Verification items for this drawing (mm, ordinates from the low corner). A direction names the side the tool comes from. Round coordinates to 2 decimals unless told otherwise and drop trailing zeros. Order: outer loops, then holes, each group sorted by start corner. A loop starts at its lowest first (then second) coordinate and runs counter-clockwise, first axis right, second up.
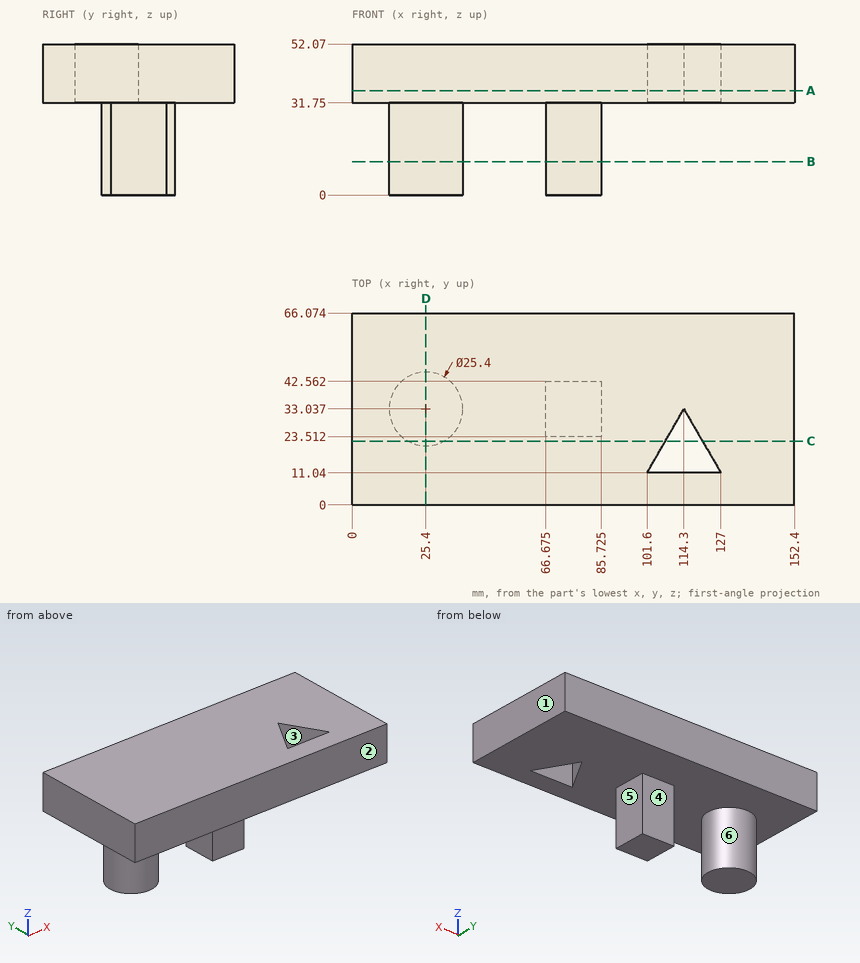
Item 1: Access from +Z, -Z, +X, -X, +Y, -Y to the whole of each face (thin tool, end or side, straight path). Record for the marked faces 4, 5 and 6.
Answer:
face 4: -Z, +X, +Y
face 5: -Z, +X, +Y, -Y
face 6: -Z
Item 2: Sectioned sample at A-A (z = 36). Record the cut outline in (x, y), and give its area (3 significant figures).
Answer:
outline: (0, 0) - (152.4, 0) - (152.4, 66.07) - (0, 66.07) - close; hole (101.6, 11.04) - (127, 11.04) - (114.3, 33.04) - close
area: 9,790 mm2
Item 3: Go/stop test with flat-tipped pins: P1, Ø9.5, axis at x = 78.5, z = 10.5, coming from the +Y side; P2, Ø10, axis at y = 47.5, z = 14.5, coming from the -X side; P3, Ø21, axis at x = 73, z = 20.5, coming from the -Y side; P4, Ø8, axis at x = 113.5, y = 23.5, coming from the +Z side. Record where each tip stops, or that it passes through.
Answer:
P1: stops at y = 42.56
P2: stops at x = 16.93
P3: stops at y = 23.51
P4: passes through
Item 4: Release check for a two-part mould opening along Y. For the marked faces 1, 2 and 3 record: released by +Y, released by -Y, zero draft, split by the parting line, or undercut.
Answer:
face 1: zero draft
face 2: released by -Y
face 3: undercut
Item 5: Scan lines: line 1 along Y through (x, z) = (77, 8.5); line 2 along Z through (x, y) = (109, 60.5); line 3 along X through (y, z) = (40, 12) (3 decimals). Record each from-to range of solid material in increasing order.
Answer:
line 1: y = 23.51 to 42.56
line 2: z = 31.75 to 52.07
line 3: x = 14.779 to 36.021, 66.675 to 85.725
Item 6: Sectioned sample at D-D (x = 25.4). Record the cut outline in (y, z).
Answer:
outline: (0, 31.75) - (20.34, 31.75) - (20.34, 0) - (45.74, 0) - (45.74, 31.75) - (66.07, 31.75) - (66.07, 52.07) - (0, 52.07) - close
Item 7: Sectioned sample at C-C (y = 22). Record the cut outline in (x, z), and give its area (3 significant figures).
Answer:
outline: (0, 31.75) - (19.12, 31.75) - (19.12, 0) - (31.68, 0) - (31.68, 31.75) - (107.93, 31.75) - (107.93, 52.07) - (0, 52.07) - close; (120.67, 31.75) - (152.4, 31.75) - (152.4, 52.07) - (120.67, 52.07) - close
area: 3,240 mm2
Item 8: Sectioned sample at B-B (z = 11.5). Record the cut outline in (x, y) (3 decimals).
Answer:
outline: circle Ø25.4 at (25.4, 33.037); (66.675, 23.512) - (85.725, 23.512) - (85.725, 42.562) - (66.675, 42.562) - close
